Input: part model. Units: mm. Frame: model coordinates. Coordinates: 2 decimals unless noted, no trailing zeros. Write each loop counter-clockwise with the first axis right and the second up, starting at its lowest first coordinate (ties: lowest second). Pieces come first, ordered by that corner, then holes. Notation, with made-up numbers: (45.25, -24.75) - (93.25, -24.75) arc R21 cw to (93.25, -13.75) - close; hole circle Ø4 at (29.5, 21.5). An arc over 180 degrees is marked (long way). Use a Markdown table: item, result. Add a question column.
Q1. Section query B-B (x = -56.5). Return the cut outline in (y, z), then the cut area to 3 significant figures.
Q2. Material intervals for probe 1 along X at (y, z) = (-1.3, -4.5); probe 2 along Z at (x, y) = (-39, -1.6); probe 3 along Z at (x, y) = (-21.5, -1.35), sorted ascending. Write a range as from..to.
Q3. Pin query (flat end, axial travel): P1, Ø0.5, axis at y = 0.5, z = -39, coming from the +X side. Return the tip coordinate at first contact, or that it passes through.
Q4. Section query A-A (z = -9.5). Return the cut outline in (x, y), then the cut area to 3 significant figures.
Q5. Section query C-C (y = 0.5). Return the cut outline in (x, z), then the cut area to 3 significant figures.
from build123d import *

# Parameters (mm, degrees)
SKETCH1_R           = 49
SKETCH1_R_2         = 41.538
BOSS_EXTRUDE1_DEPTH = 1
CUT_EXTRUDE1_START  = -10
CUT_EXTRUDE1_DEPTH  = 10
CUT_EXTRUDE2_DEPTH  = 10
BOSS_EXTRUDE2_START = 2
SKETCH4_R           = 49
SKETCH4_R_2         = 42.55
BOSS_EXTRUDE2_DEPTH = 2
SKETCH5_R           = 1.7
CUT_EXTRUDE3_DEPTH  = 95.04770922


with BuildPart() as part:
    # Sketch1 → Boss-Extrude1 (new body)
    with BuildSketch(Plane(origin=(0, 0, 0), x_dir=(1, 0, 0), z_dir=(0, 1, 0))):
        with Locations(Location((-17.234280104, -2.988648948, 0), (0, 0, 270))):
            Circle(SKETCH1_R)
        with Locations(Location((-17.234280104, -2.988648948, 0), (0, 0, 270))):
            Circle(SKETCH1_R_2, mode=Mode.SUBTRACT)
    extrude(amount=BOSS_EXTRUDE1_DEPTH)

    # Sketch2 → Cut-Extrude1 (cut)
    with BuildSketch(Plane(origin=(0, 1, 0), x_dir=(1, 0, 0), z_dir=(0, 1, 0)).offset(CUT_EXTRUDE1_START)):
        with BuildLine():
            Line((-16.734280104, 38.54634165), (-16.734280104, 39.546412401))
            ThreePointArc((-16.734280104, 39.546412401), (-17.234280104, 39.549351052), (-17.734280104, 39.546412401))
            Line((-17.734280104, 39.546412401), (-17.734280104, 38.54634165))
            ThreePointArc((-17.734280104, 38.54634165), (-17.234280104, 38.549351052), (-16.734280104, 38.54634165))
        make_face()
    extrude(amount=CUT_EXTRUDE1_DEPTH, mode=Mode.SUBTRACT)

    # Sketch3 → Cut-Extrude2 (cut)
    with BuildSketch(Plane.XZ):
        with BuildLine():
            Line((-17.734280104, -38.54634165), (-17.734280104, -39.55841323))
            ThreePointArc((-17.734280104, -39.55841323), (-17.234280104, -39.561351052), (-16.734280104, -39.55841323))
            Line((-16.734280104, -39.55841323), (-16.734280104, -38.54634165))
            ThreePointArc((-16.734280104, -38.54634165), (-17.234280104, -38.549351052), (-17.734280104, -38.54634165))
        make_face()
    extrude(amount=-CUT_EXTRUDE2_DEPTH, mode=Mode.SUBTRACT)

    # Sketch4 → Boss-Extrude2 (add)
    with BuildSketch(Plane.XZ.offset(BOSS_EXTRUDE2_START)):
        with Locations(Location((-17.234280104, 2.988648948, 0), (0, 0, 270))):
            Circle(SKETCH4_R)
        with Locations(Location((-17.234280104, 2.988648948, 0), (0, 0, 270))):
            Circle(SKETCH4_R_2, mode=Mode.SUBTRACT)
    extrude(amount=-BOSS_EXTRUDE2_DEPTH)

    # Sketch5 → Cut-Extrude3 (cut, through all)
    with BuildSketch(Plane(origin=(12.15729015, 4, 5.600017102), x_dir=(1, 0, 0), z_dir=(0, 1, 0))):
        with Locations(Location((-29.391570254, 48.111368154, 0), (0, 0, 180))):
            Circle(SKETCH5_R)
        with Locations(Location((-74.200323016, 10.512360238, 0), (0, 0, 180))):
            Circle(SKETCH5_R)
        with Locations(Location((-52.141570254, -36.792787718, 0), (0, 0, 180))):
            Circle(SKETCH5_R)
        with Locations(Location((-6.641570254, -36.792787718, 0), (0, 0, 180))):
            Circle(SKETCH5_R)
        with Locations(Location((15.417182508, 10.512360238, 0), (0, 0, 180))):
            Circle(SKETCH5_R)
    extrude(amount=-CUT_EXTRUDE3_DEPTH, mode=Mode.SUBTRACT)


solid = part.part
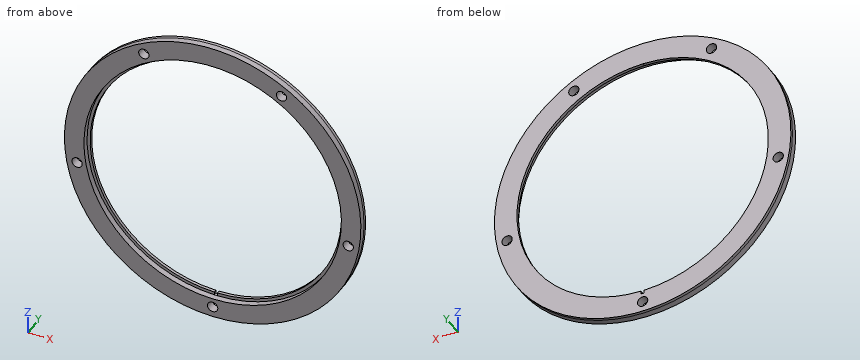
Values follow:
| question | item | result |
|---|---|---|
| 1 | outline | (-2, -26.32) - (1, -26.32) - (1, -10.56) - (0, -10.56) - (0, -13.4) - (-2, -13.4) - close; (-2, 19.38) - (0, 19.38) - (0, 16.54) - (1, 16.54) - (1, 32.3) - (-2, 32.3) - close |
| 1 | area | 83.2 mm2 |
| 2 | probe 1 | -65.66..-63.69, -60.39..-59.12, 24.65..25.93, 29.22..31.19 |
| 2 | probe 2 | -40.91..-33.57, 39.55..41.01, 43.78..46.89 |
| 2 | probe 3 | -45.83..-39.35, 45.32..51.8 |
| 3 | P1 | x = 8.43 |
| 4 | outline | (-64.62, -2) - (-57.91, -2) - (-57.91, 0) - (-56.85, 0) - (-56.85, 1) - (-64.62, 1) - close; (22.38, 0) - (23.44, 0) - (23.44, -2) - (30.15, -2) - (30.15, 1) - (22.38, 1) - close |
| 4 | area | 42.4 mm2 |
| 5 | outline | circle Ø98 at (-17.23, 2.99); hole circle Ø3.4 at (-62.04, -4.91); hole circle Ø3.4 at (-39.98, 42.39); hole circle Ø3.4 at (-17.23, -42.51); hole (-17.73, -39.56) arc R42.55 ccw to (-16.73, -39.56) - (-16.73, -38.55) arc R41.54 ccw (long way) to (-17.73, -38.55) - close; hole circle Ø3.4 at (5.52, 42.39); hole circle Ø3.4 at (27.57, -4.91) |
| 5 | area | 2,080 mm2 |
